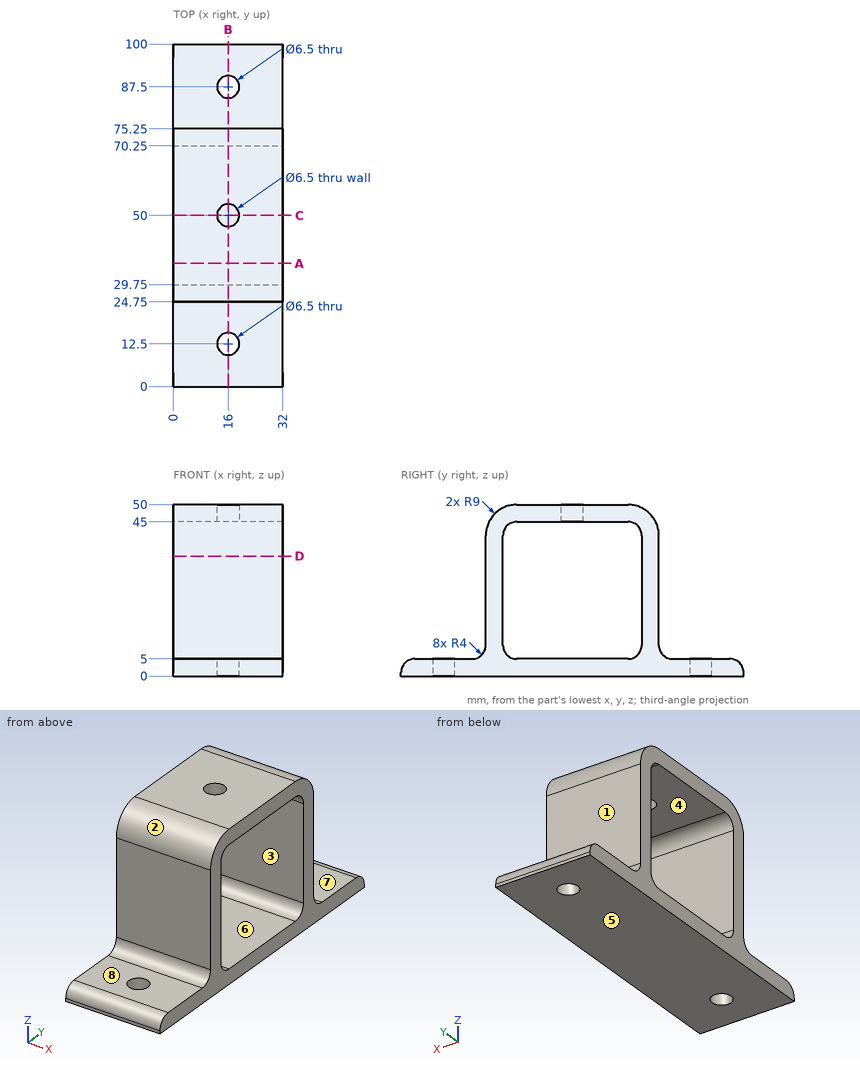
Geometry check sheet. Reference: drawing and pictorial views, mm from the part's lowest x, y, z. A direction names the side the tool comes from. Round coordinates to 2 decimals unless told otherwise and drop trailing zeros. Loops run counter-clockwise (first coordinate to the right, second up) from the corner with the lowest first, then second, coordinate; pieces in that order, holes last. Notation, with made-up numbers: (42.25, 62) -> (47.25, 62) arc R19 cw to (47.25, 73) -> close; hole circle Ø10 at (20, -32). An arc over 180 degrees is marked (long way). Answer as a JSON object with one key per item and string values. Group by question number.
Item 1: Release check for a two-part mould opening along Z. For the marked faces 1, 2, 3 and 4 record: pulls with the +Z half, pulls with the -Z half, needs draft (parallel to the pull), parting line crosses it, or undercut.
Item 2: Cross-section at C-C, the plane y = 50. Record the cut outline in (x, z).
Item 3: Depth check by flat-ended pin: pin 1 Ø13.5 at (x, y) = (8, 11) entering from +Z; pin 2 Ø10 at (x, z) = (28, 44) entering from -Y; pin 3 Ø10 at (y, z) = (16.5, 5.5) entering from +X; pin 4 Ø1 at (x, z) = (16.5, 8.5) entering from +Y. Enter the tip coordinate at first touch or a pass-through.
Item 4: Cross-section at D-D, the plane z = 35. Record the cut outline in (x, y).
Item 5: Cross-section at A-A, the plane y = 36. Record the cut outline in (x, z).
Item 6: Thickness scan on line 1 along Z through (x, y) = (5.5, 55.5); line 2 along Y through (x, z) = (2, 38); line 3 along X through (y, z) = (12.5, 3.1). Record the ranges inside material, lowest first.
Item 7: Set-up check for the marked faces 5, 6, 7 and 8: record each of +Z, -Z, +X, -X, +Y, -Y from which the full face is reachable in a straight line by a thin tool's end or side.
Item 8: Cross-section at B-B, the plane x = 16. Count the separate pieces of the cut face and the enclosed holes in it, plus the area to 3 significant figures.
Determined:
{
 "1": {"face 1": "needs draft", "face 2": "pulls with the +Z half", "face 3": "undercut", "face 4": "undercut"},
 "2": {"outline": "(0, 0) -> (32, 0) -> (32, 5) -> (0, 5) -> close; (0, 45) -> (12.75, 45) -> (12.75, 50) -> (0, 50) -> close; (19.25, 45) -> (32, 45) -> (32, 50) -> (19.25, 50) -> close"},
 "3": {"pin 1": "stops at z = 5", "pin 2": "stops at y = 24.75", "pin 3": "stops at x = 32", "pin 4": "stops at y = 75.38"},
 "4": {"outline": "(0, 24.75) -> (32, 24.75) -> (32, 29.75) -> (0, 29.75) -> close; (0, 70.25) -> (32, 70.25) -> (32, 75.25) -> (0, 75.25) -> close"},
 "5": {"outline": "(0, 0) -> (32, 0) -> (32, 5) -> (0, 5) -> close; (0, 45) -> (32, 45) -> (32, 50) -> (0, 50) -> close"},
 "6": {"line 1": "z = 0 to 5, 45 to 50", "line 2": "y = 24.75 to 29.75, 70.25 to 75.25", "line 3": "x = 0 to 12.75, 19.25 to 32"},
 "7": {"face 5": "-Z, +X, -X, +Y, -Y", "face 6": "+X, -X", "face 7": "+Z, +X, -X, +Y", "face 8": "+Z, +X, -X, -Y"},
 "8": {"separate pieces": "3", "enclosed holes": "0", "area": "1,030 mm²"}
}
